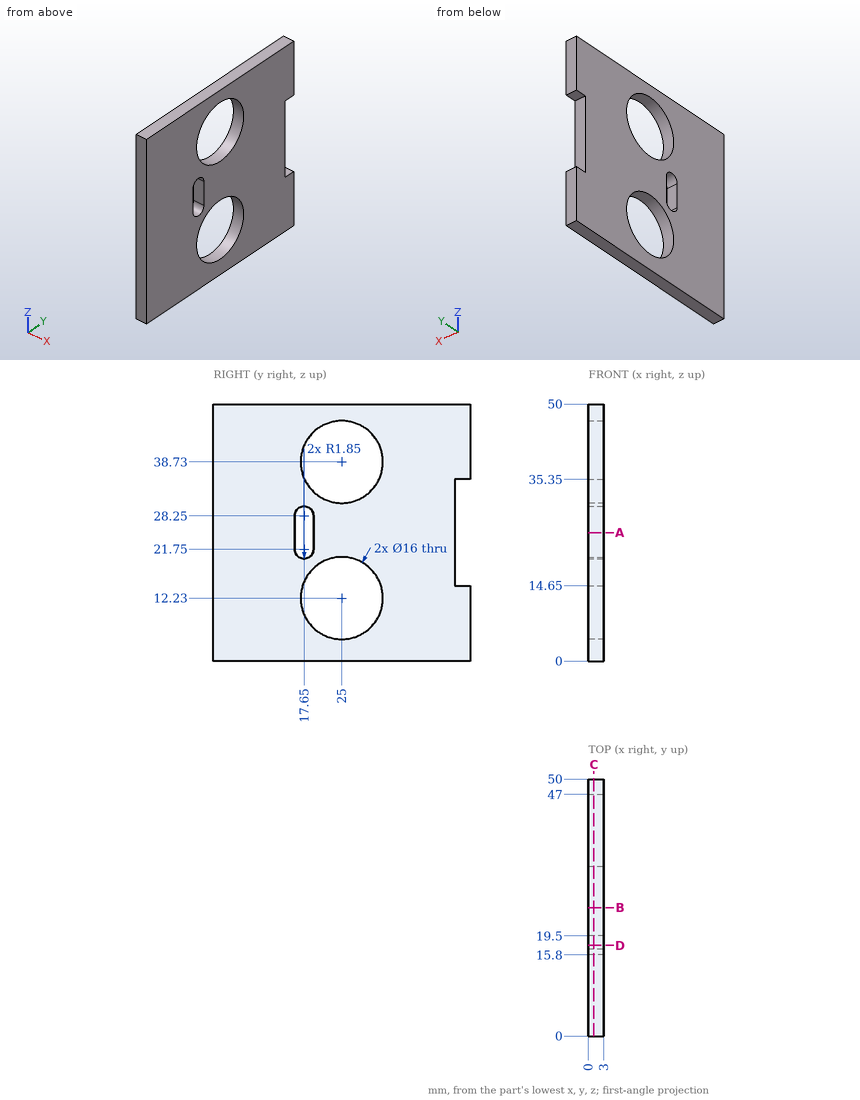
Study the drawing (mm; zero at the part's minimum x, y, z) and answer. Round coordinates to 2 decimals unless told otherwise and drop trailing zeros. Write each loop counter-clockwise with the first axis right and the second up, starting at its lowest first coordinate (ties: lowest second). Pieces come first, ordered by that corner, then holes. Notation, with made-up numbers: (4, -2) - (13, -2) arc R15 cw to (13, 13) - close; hole circle Ø1 at (35.5, 25.5). An arc over 180 degrees is marked (long way). Use a Markdown table: item, result. Add a question column.
1. Flat-ended cylindrical pins translate along their axes: P1, Ø6, axis at y = 19.5, z = 37, coming from the +X side; P2, Ø9.5, axis at y = 25, z = 12.23, coming from the +X side; P3, Ø0.9, axis at x = 2, z = 24, coming from the +Y side. Find the tip coordinate at first contact, or state that the pin passes through.
2. The part is cut by section C-C (x = 1.1). Write down the section's boundary in (y, z).
3. The part is cut by section A-A (z = 25). Write down the section's boundary in (x, y), and give its area (3 significant figures).
4. The part is cut by section D-D (y = 17.65). Write down the section's boundary in (x, z), and give its area (3 significant figures).
5. The part is cut by section B-B (y = 25). Write down the section's boundary in (x, z).
6. Consider line 1 (Y direction, x = 2.2, z = 38.73); line 2 (Z direction, x = 1.15, y = 30) (3 decimals); line 3 (Y direction, x = 0.8, z = 24.5). Determine where each line is inside the solid, lowest interval first.
Reported:
| question | item | result |
|---|---|---|
| 1 | P1 | x = 3 |
| 1 | P2 | through |
| 1 | P3 | y = 47 |
| 2 | outline | (0, 0) - (50, 0) - (50, 14.65) - (47, 14.65) - (47, 35.35) - (50, 35.35) - (50, 50) - (0, 50) - close; hole (15.8, 21.75) arc R1.85 ccw to (19.5, 21.75) - (19.5, 28.25) arc R1.85 ccw to (15.8, 28.25) - close; hole circle Ø16 at (25, 12.23); hole circle Ø16 at (25, 38.73) |
| 3 | outline | (0, 0) - (3, 0) - (3, 15.8) - (0, 15.8) - close; (0, 19.5) - (3, 19.5) - (3, 47) - (0, 47) - close |
| 3 | area | 130 mm^2 |
| 4 | outline | (0, 0) - (3, 0) - (3, 9.07) - (0, 9.07) - close; (0, 15.39) - (3, 15.39) - (3, 19.9) - (0, 19.9) - close; (0, 30.1) - (3, 30.1) - (3, 35.57) - (0, 35.57) - close; (0, 41.89) - (3, 41.89) - (3, 50) - (0, 50) - close |
| 4 | area | 81.5 mm^2 |
| 5 | outline | (0, 0) - (3, 0) - (3, 4.23) - (0, 4.23) - close; (0, 20.23) - (3, 20.23) - (3, 30.73) - (0, 30.73) - close; (0, 46.73) - (3, 46.73) - (3, 50) - (0, 50) - close |
| 6 | line 1 | 0 to 17, 33 to 50 |
| 6 | line 2 | 0 to 5.985, 18.475 to 32.485, 44.975 to 50 |
| 6 | line 3 | 0 to 15.8, 19.5 to 47 |
